```python
from build123d import *

# Parameters (mm, degrees)
BOSS_EXTRU_1_DEPTH = 2
ESQUISSE3_W        = 4
ESQUISSE3_H        = 4
BOSS_EXTRU_2_DEPTH = 20
ESQUISSE4_W        = 4
ESQUISSE4_H        = 4
BOSS_EXTRU_3_DEPTH = 10
ESQUISSE5_R        = 4.435199719
ESQUISSE5_R_2      = 4
BOSS_EXTRU_4_DEPTH = 2


with BuildPart() as part:
    # Esquisse1 → Boss.-Extru.1 (new body, symmetric)
    with BuildSketch(Plane.XY):
        Polygon((0, 0), (0, 50), (44, 50), (44, 100), (46, 100), (46, 48), (2, 48), (2, 0), align=None)
    boss_extru_1 = extrude(amount=BOSS_EXTRU_1_DEPTH, both=True)

    # Esquisse2 → Révolution1 (revolve)
    with BuildSketch(Plane.XY):
        with BuildLine():
            Line((43.480681174, 107.464101615), (43.230681174, 107.897114317))
            ThreePointArc((43.230681174, 107.897114317), (47.730681174, 107.897114317), (49.980681174, 104))
            Line((49.980681174, 104), (49.480681174, 104))
            ThreePointArc((49.480681174, 104), (47.480681174, 107.464101615), (43.480681174, 107.464101615))
        make_face()
    revolve(axis=Axis((49.980681174, 104, 0), (-1, 0, 0)))

    # Symétrie1: Boss.-Extru.1 across plane
    add(boss_extru_1.mirror(Plane(origin=(0, 0, -2), x_dir=(0, 0, 1), z_dir=(-1, 0, 0))))

    # Esquisse3 → Boss.-Extru.2 (add)
    with BuildSketch(Plane.XY):
        with Locations((0, -2)):
            Rectangle(ESQUISSE3_W, ESQUISSE3_H)
    boss_extru_2 = extrude(amount=BOSS_EXTRU_2_DEPTH)

    # Esquisse4 → Boss.-Extru.3 (add)
    with BuildSketch(Plane(origin=(0, -4, 0), x_dir=(-1, 0, 0), z_dir=(0, -1, 0))):
        with Locations((0, -18)):
            Rectangle(ESQUISSE4_W, ESQUISSE4_H)
    boss_extru_3 = extrude(amount=BOSS_EXTRU_3_DEPTH)

    # Symétrie2: Boss.-Extru.2, Boss.-Extru.3 across plane
    add(boss_extru_2.mirror(Plane(origin=(0, 0, 0), x_dir=(1, 0, 0), z_dir=(0, 0, -1))))
    add(boss_extru_3.mirror(Plane(origin=(0, 0, 0), x_dir=(1, 0, 0), z_dir=(0, 0, -1))))

    # Esquisse5 → Boss.-Extru.4 (add)
    with BuildSketch(Plane.ZY.offset(46)):
        with Locations((0, 103.958660954)):
            Circle(ESQUISSE5_R)
        with Locations((0, 103.958660954)):
            Circle(ESQUISSE5_R_2, mode=Mode.SUBTRACT)
    extrude(amount=-BOSS_EXTRU_4_DEPTH)


solid = part.part
```
Design review of the part built by this model. Coordinates are the model's own, in mm. A direction names the side the tool comes from. Coordinates: 2 decimals unless noted, no trailing zeros. Loops run counter-clockwise (first coordinate to the right, second up) from the corner with the lowest first, then second, coordinate; pieces in that order, holes last. Notation, with made-up numbers: (70, 47.5) -> (88, 47.5) arc R21 ccw to (88, 79.5) -> close; hole circle Ø11 at (31, 57). An arc over 180 degrees is marked (long way). Answer as a JSON object with one key per item and string values.
Q1. To check wall thickness, follow L1, parallel to X at y = 64, z = -1.5; L2, parallel to X at y = -3, z = -9.5. State the ranges of each line that lie inside material, in increasing order.
Answer block:
{"L1": "x = -46 to -44, 44 to 46", "L2": "x = -2 to 2"}
Q2. Tool access review of faces 4 (the flat face through (-44, 80, 0)), 5 (the flat face through (0, 47, 2)), 6 (the cylindrical face through (-45.014, 107.955, 0.168)), 7 (the flat face through (-2, 8, 0)), 8 (the flat face through (46, 74, 0)): name each direction out of +Z, -Z, +X, -X, +Y, -Y from which nothing blocks a thin tool from reaching the whole face with its end or side.
Answer block:
{"face 4": "+Z, -Z, +Y", "face 5": "+Z, +X, -X", "face 6": "-X", "face 7": "+Z, -Z, -X, -Y", "face 8": "+Z, -Z, +X, -Y"}
Q3. Take a section at C-C on z = -8. Give the boundary of the cut face in (x, y).
Answer block:
{"outline": "(-2, -4) -> (2, -4) -> (2, 0) -> (-2, 0) -> close"}
Q4. Clearance check with flat-ended pins moving along their axes: pin 1 Ø12 at (y, z) = (25.5, -3.5) entering from +X; pin 2 Ø0.6 at (x, z) = (44.5, 2) entering from +Y; pin 3 Ø8 at (x, z) = (16.5, 0.5) entering from +Y; pin 4 Ø1.5 at (x, z) = (-35.5, 4.5) entering from -Y. State where each tip first meets the part, or that it passes through.
Answer block:
{"pin 1": "stops at x = 2", "pin 2": "stops at y = 108.07", "pin 3": "stops at y = 50", "pin 4": "passes through"}
Q5. The part is to be moulded in two halves that separate along Z. For faces 1 (the flat face through (0, 0, 11)), 2 (the flat face through (0, -4, 0)), 3 (the cylindrical face through (-45.01, 108.39, 0.17)), say which applies: +Z half, -Z half, draft (parallel to the pull), parting line (faces both ways), or undercut.
Answer block:
{"face 1": "draft", "face 2": "undercut", "face 3": "parting line"}
Q6. Take a section at A-A on y = 79. Give the boundary of the cut face in (x, z).
Answer block:
{"outline": "(-46, -2) -> (-44, -2) -> (-44, 2) -> (-46, 2) -> close; (44, -2) -> (46, -2) -> (46, 2) -> (44, 2) -> close"}
Q7. Take a section at D-D on x = 5.5. Give the boundary of the cut face in (y, z), plus the area to 3 significant figures.
Answer block:
{"outline": "(48, -2) -> (50, -2) -> (50, 2) -> (48, 2) -> close", "area": "8.00 mm^2"}
Q8. Take a section at B-B on y = 104. Give the boundary of the cut face in (x, z) (3 decimals), plus the area to 3 significant figures.
Answer block:
{"outline": "(-46, -4.435) -> (-44, -4.435) -> (-44, -4) -> (-46, -4) -> close; (-46, 4) -> (-44, 4) -> (-44, 4.435) -> (-46, 4.435) -> close; (43.231, -3.897) arc R4.5 ccw (long way) to (43.231, 3.897) -> (43.481, 3.464) arc R4 cw (long way) to (43.481, -3.464) -> close", "area": "10.6 mm^2"}
